from build123d import *

# Parameters (mm, degrees)
SKETCH1_W           = 101.6
SKETCH1_H           = 101.6
BOSS_EXTRUDE1_DEPTH = 10
SKETCH2_R           = 5
CUT_EXTRUDE1_DEPTH  = 5
SKETCH3_R           = 12.5
BOSS_EXTRUDE2_DEPTH = 2
SKETCH4_R           = 7.75
BOSS_EXTRUDE3_DEPTH = 50
SKETCH6_W           = 101.6
SKETCH6_H           = 101.6
CUT_EXTRUDE2_DEPTH  = 10
SKETCH7_R           = 7.023915829
CUT_EXTRUDE3_DEPTH  = 30


with BuildPart() as part:
    # Sketch1 → Boss-Extrude1 (new body)
    with BuildSketch(Plane(origin=(0, 0, 0), x_dir=(1, 0, 0), z_dir=(0, 1, 0))):
        Rectangle(SKETCH1_W, SKETCH1_H)
    extrude(amount=BOSS_EXTRUDE1_DEPTH)

    # Sketch2 → Cut-Extrude1 (cut)
    with BuildSketch(Plane(origin=(0, 0, 0), x_dir=(-1, 0, 0), z_dir=(0, -1, 0))):
        with Locations(Location((0, 0, 0), (0, 0, 90))):
            Circle(SKETCH2_R)
    extrude(amount=-CUT_EXTRUDE1_DEPTH, mode=Mode.SUBTRACT)

    # Sketch3 → Boss-Extrude2 (add)
    with BuildSketch(Plane(origin=(0, 10, 0), x_dir=(1, 0, 0), z_dir=(0, 1, 0))):
        with Locations(Location((0, 0, 0), (0, 0, 90))):
            Circle(SKETCH3_R)
    extrude(amount=BOSS_EXTRUDE2_DEPTH)

    # Sketch4 → Boss-Extrude3 (add)
    with BuildSketch(Plane(origin=(0, 12, 0), x_dir=(1, 0, 0), z_dir=(0, 1, 0))):
        with Locations(Location((0, 0, 0), (0, 0, 270))):
            Circle(SKETCH4_R)
    extrude(amount=BOSS_EXTRUDE3_DEPTH)

    # Sketch6 → Cut-Extrude2 (cut)
    with BuildSketch(Plane(origin=(0, 10, 0), x_dir=(1, 0, 0), z_dir=(0, 1, 0))):
        Rectangle(SKETCH6_W, SKETCH6_H)
    extrude(amount=-CUT_EXTRUDE2_DEPTH, mode=Mode.SUBTRACT)

    # Sketch7 → Cut-Extrude3 (cut)
    with BuildSketch(Plane(origin=(0, 62, 0), x_dir=(1, 0, 0), z_dir=(0, 1, 0))):
        with Locations(Location((0, 0, 0), (0, 0, 270))):
            Circle(SKETCH7_R)
    extrude(amount=-CUT_EXTRUDE3_DEPTH, mode=Mode.SUBTRACT)


solid = part.part
The listing builds one solid part. Answer for the finished solid, in the listing's coordinates (mm). A direction names the side the tool comes from. Give positions to 0.01 mm unless a question says otherwise; leave off trailing zeros. Loops run counter-clockwise (first coordinate to the right, second up) from the corner with the lowest first, then second, coordinate; pieces in that order, holes last.
Item 1: A cutting plane is placed at B-B (x = 0). Give the vertices of the cut face in (y, z).
Derived:
outline: (10, -12.5) - (12, -12.5) - (12, -7.75) - (62, -7.75) - (62, -7.02) - (32, -7.02) - (32, 7.02) - (62, 7.02) - (62, 7.75) - (12, 7.75) - (12, 12.5) - (10, 12.5) - close
Item 2: A cutting plane is placed at A-A (z = 0). Give the vertices of the cut face in (x, y).
Derived:
outline: (-12.5, 10) - (12.5, 10) - (12.5, 12) - (7.75, 12) - (7.75, 62) - (7.02, 62) - (7.02, 32) - (-7.02, 32) - (-7.02, 62) - (-7.75, 62) - (-7.75, 12) - (-12.5, 12) - close
Item 3: A cutting plane is placed at D-D (y = 21). Give the vertices of the cut face in (x, z), then the cut area to 3 significant figures.
Derived:
outline: circle Ø15.5 at (0, 0)
area: 189 mm2
Item 4: Determine the mould class of faces 1 (the flat face through (4, 62, -6)), 2 (the flat face through (0, 32, 0)), 3 (the cylindrical face through (-3.755, 10.986, -11.923)) for opening direction Z: +Z half, -Z half, draft (parallel to the pull), parting line (faces both ways), or undercut.
Derived:
face 1: draft
face 2: undercut
face 3: parting line
Item 5: Find the intervals of material crossed by line 1 along Z through (x, y) = (-0.25, 49.5); line 2 along Y through (x, z) = (6, -6.25), in increasing order.
Derived:
line 1: z = -7.75 to -7.02, 7.02 to 7.75
line 2: y = 10 to 12
Item 6: A cutting plane is placed at C-C (y = 38). Give the vertices of the cut face in (x, z).
Derived:
outline: circle Ø15.5 at (0, 0); hole circle Ø14.05 at (0, 0)
Item 7: Each of these flat-tipped pins is pushed along its axis until it touches: pin 1 Ø4 at (y, z) = (20, 3) entering from -X; pin 2 Ø2 at (x, y) = (2.5, 30.5) entering from -Z; pin 3 Ø1.5 at (y, z) = (22, -4.5) entering from -X; pin 4 Ø3 at (y, z) = (54, 9.5) entering from +X. Where does it stop, or does it pass through?
Derived:
pin 1: stops at x = -7.69
pin 2: stops at z = -7.6
pin 3: stops at x = -6.78
pin 4: passes through
Item 8: A tool of negligible diameter and unlimited length cuts with its end or side. For faces 4 (the flat face through (8, 12, 0)), 5 (the flat face through (0, 10, 0)), from which of +Z, -Z, +X, -X, +Y, -Y can it reach the whole face along a straight path? Write none if from no direction.
Derived:
face 4: +Y
face 5: +Z, -Z, +X, -X, -Y
